For this review, take the finished solid that the model builds, in its own axes (mm). A direction names the side the tool comes from. Round coordinates to 2 decimals unless told otherwise and drop trailing zeros. Order: outer loops, then holes, each group sorted by start corner. A loop starts at its lowest first (then second) coordinate and runs counter-clockwise, first axis right, second up.
```python
from build123d import *

# Parameters (mm, degrees)
SKETCH1_W               = 48
SKETCH1_H               = 45
SKETCH1_R               = 2.15
BOSS_EXTRUDE1_DEPTH     = 5
CUT_EXTRUDE1_DEPTH      = 66.984846745
CUT_EXTRUDE1_DEPTH_BACK = 66.984846745
FILLET1_R               = 5
CHAMFER1_SIZE           = 2.3


with BuildPart() as part:
    # Sketch1 → Boss-Extrude1 (new body)
    with BuildSketch(Plane(origin=(0, 0, 0), x_dir=(1, 0, 0), z_dir=(0, 1, 0))):
        with Locations((-24, 22.5)):
            Rectangle(SKETCH1_W, SKETCH1_H)
        with Locations(Location((-40, 3, 0), (0, 0, 270))):
            Circle(SKETCH1_R, mode=Mode.SUBTRACT)
        with Locations(Location((-8, 3, 0), (0, 0, 270))):
            Circle(SKETCH1_R, mode=Mode.SUBTRACT)
        with BuildLine():
            Line((-30, 10.75), (-5, 10.75))
            ThreePointArc((-5, 10.75), (-3.25, 9), (-5, 7.25))
            Line((-5, 7.25), (-30, 7.25))
            ThreePointArc((-30, 7.25), (-31.75, 9), (-30, 10.75))
        make_face(mode=Mode.SUBTRACT)
        with BuildLine():
            Line((-30, 42.75), (-5, 42.75))
            ThreePointArc((-5, 42.75), (-3.25, 41), (-5, 39.25))
            Line((-5, 39.25), (-30, 39.25))
            ThreePointArc((-30, 39.25), (-31.75, 41), (-30, 42.75))
        make_face(mode=Mode.SUBTRACT)
    extrude(amount=BOSS_EXTRUDE1_DEPTH)

    # Sketch2 → Cut-Extrude1 (cut, two sides: drawn at the far end of the back side and taken through both)
    with BuildSketch(Plane(origin=(0, 5, 0), x_dir=(1, 0, 0), z_dir=(0, 1, 0)).offset(-CUT_EXTRUDE1_DEPTH_BACK)):
        Polygon((-31.732050808, 45), (-48, 16.823085464), (-48, 45), align=None)
    extrude(amount=CUT_EXTRUDE1_DEPTH + CUT_EXTRUDE1_DEPTH_BACK, mode=Mode.SUBTRACT)

    # Fillet1
    fillet1_edges = [part.edges().sort_by_distance(p)[0] for p in [
        (-31.732050808, 2.5, -45),
        (-48, 2.5, -16.823085464),
        (0, 2.5, 0),
        (-48, 2.5, 0),
        (0, 2.5, -45),
    ]]
    fillet(fillet1_edges, radius=FILLET1_R)

    # Chamfer1
    # the kernel refuses this chamfer: 2.3 mm, written as the material it takes off along each edge
    with BuildSketch(Plane(origin=(-40, 5, -3), x_dir=(0, 0, 1), z_dir=(-1, 0, 0))) as chamfer1_piece_1:
        Polygon((2.15 + CHAMFER1_SIZE, 0), (2.15, -CHAMFER1_SIZE), (2.15, 0), align=None)
    revolve(axis=Axis((-40, 5, -3), (0, 1, 0)), mode=Mode.SUBTRACT)
    with BuildSketch(Plane(origin=(-8, 5, -3), x_dir=(0, 0, 1), z_dir=(-1, 0, 0))) as chamfer1_piece_2:
        Polygon((2.15 + CHAMFER1_SIZE, 0), (2.15, -CHAMFER1_SIZE), (2.15, 0), align=None)
    revolve(axis=Axis((-8, 5, -3), (0, 1, 0)), mode=Mode.SUBTRACT)


solid = part.part
```
Q1. Take a section at C-C, the plane y = 1.75. State the section outline as (x, z) points, plus the area to 3 significant figures.
Q2. Clearance check with flat-ended pins moving along their axes: pin 1 (7 mm diameter, centred on x = -40, z = -3, fed in from -Y); pin 2 (2 mm diameter, centred on y = 3, z = -33, fed in from -X). State where each tip first meets the part, or that it passes through.
Q3. Take a section at A-A, the plane x = -19. State the section outline as (y, z) points, plus the area to 3 significant figures.
Q4. Take a section at B-B, the plane x = -8. State the section outline as (y, z) points.
Q5. Wall thickness on line 1 (Z direction, x = -19, y = 0.75); line 2 (X direction, y = 2.75, z = -9); line 3 (X direction, y = 1.5, z = -3): over which ranges is each line inside the solid? List them lowest first.
Q6. Tool access review of faces 1 (the face through (-3.25, 2.46, -41.04)), 2 (the face through (-31.4, 2.5, -44.3)): name each direction out of +Z, -Z, +X, -X, +Y, -Y from which nothing blocks a thin tool from reaching the whole face with its end or side.
Q7. Mouldability with a two-part tool opening along Z and no side actions: class faces 3 (the face through (-17, 2, -7.25)), 4 (the face through (-40.154, 2.465, -30.413)), 5 (the face through (-2, 3, -1)), 6 (the face through (-3.25, 2.46, -9.04)) as +Z half, -Z half, draft (parallel to the pull), parting line (faces both ways), or undercut.
Q8. Take a section at D-D, the plane z = -41. State the section outline as (x, y) points.
Working result:
1. outline: (-48, -15.48) arc R5 ccw to (-47.33, -17.98) - (-33.18, -42.5) arc R5 ccw to (-28.85, -45) - (-5, -45) arc R5 ccw to (0, -40) - (0, -5) arc R5 ccw to (-5, 0) - (-43, 0) arc R5 ccw to (-48, -5) - close; hole circle Ø4.3 at (-40, -3); hole (-30, -42.75) - (-5, -42.75) arc R1.75 ccw to (-5, -39.25) - (-30, -39.25) arc R1.75 ccw to start; hole (-30, -10.75) - (-5, -10.75) arc R1.75 ccw to (-5, -7.25) - (-30, -7.25) arc R1.75 ccw to start; hole circle Ø4.3 at (-8, -3)
1. area: 1,690 mm2
2. pin 1: stops at y = 0
2. pin 2: stops at x = -39.24
3. outline: (0, -45) - (5, -45) - (5, -42.75) - (0, -42.75) - close; (0, -39.25) - (5, -39.25) - (5, -10.75) - (0, -10.75) - close; (0, -7.25) - (5, -7.25) - (5, 0) - (0, 0) - close
3. area: 190 mm2
4. outline: (0, -45) - (5, -45) - (5, -42.75) - (0, -42.75) - close; (0, -39.25) - (5, -39.25) - (5, -10.75) - (0, -10.75) - close; (0, -7.25) - (4.8, -7.25) - (2.7, -5.15) - (0, -5.15) - close; (0, -0.85) - (2.7, -0.85) - (3.55, 0) - (0, 0) - close
5. line 1: z = -45 to -42.75, -39.25 to -10.75, -7.25 to 0
5. line 2: x = -48 to -31.75, -3.25 to 0
5. line 3: x = -47.58 to -42.15, -37.85 to -10.15, -5.85 to -0.42
6. face 1: +Y, -Y
6. face 2: -Z, -X, +Y, -Y
7. face 3: undercut
7. face 4: -Z half
7. face 5: +Z half
7. face 6: undercut
8. outline: (-34.04, 0) - (-31.75, 0) - (-31.75, 5) - (-34.04, 5) - close; (-3.25, 0) - (-0.1, 0) - (-0.1, 5) - (-3.25, 5) - close
